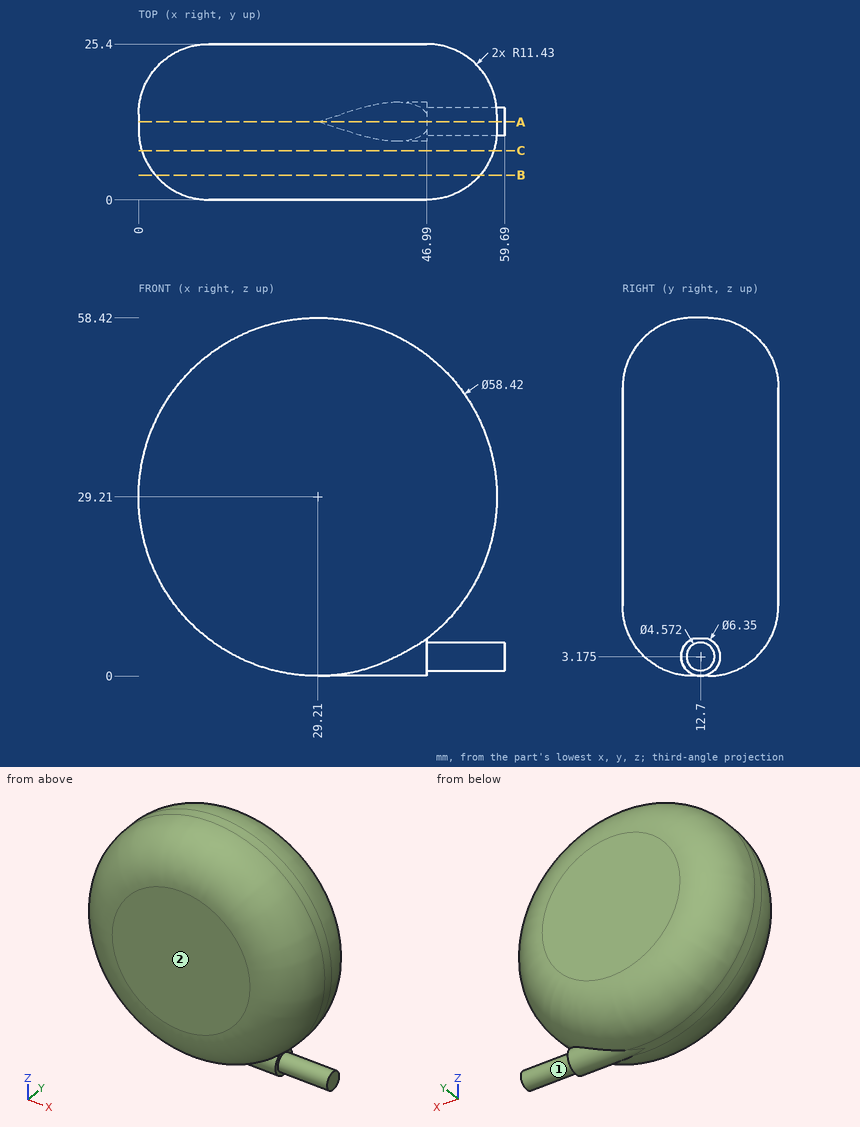
Part print with two shaded views. Sizes in mm from the minimum x, y, z corner. Give positions to 0.01 mm unless a question says otherwise; leave off trailing zeros. Order: outer loops, then holes, each group sorted by start corner. A loop starts at its lowest first (then second) coordinate and runs counter-clockwise, first axis right, second up. Notation, with made-up numbers: (-12.5, 3.25) - (21.5, 3.25) arc R16 cw to (21.5, 14.25) - close; hole circle Ø1 at (58, 16). An arc over 180 degrees is marked (long way). Write each question's results on one line, items separated by ' | '.
1. Saw through at A-A on y = 12.7. List the corners of the cut face in (x, z).
Calculated:
outline: (29.21, 0) - (46.99, 0) - (46.99, 0.89) - (59.69, 0.89) - (59.69, 5.46) - (46.99, 5.46) - (46.99, 6.03) arc R29.21 ccw (long way) to start
2. Saw through at C-C on y = 8. List the corners of the cut face in (x, z), and give its area (3 significant figures).
Calculated:
outline: circle Ø57.37 at (29.21, 29.21) | area: 2,580 mm2
3. Probe L1, parallel to Z at x = 9.5, y = 20.5; L2, parallel to Y at x = 32.5, z = 48.5; L3, parallel to Y at x = 25.5, z = 51. List the from-to ranges inside material, lowest first. Write a range as from..to.
Calculated:
L1: z = 10.52..47.9 | L2: y = 0.14..25.26 | L3: y = 0.85..24.55
4. Saw through at B-B on y = 4. List the corners of the cut face in (x, z), and give its area (3 significant figures).
Calculated:
outline: circle Ø52.93 at (29.21, 29.21) | area: 2,200 mm2
5. Pin check, flat tips, straight feed: pin 1 (4 mm diameter, centred on x = 32, y = 10, fed in from +Z); pin 2 (8 mm diameter, centred on y = 13, z = 47.5, fed in from -X); pin 3 (1 mm diameter, centred on y = 6, z = 41, fed in from -X). Stop position of each tip, or through.
Calculated:
pin 1: stops at z = 58.39 | pin 2: stops at x = 3.73 | pin 3: stops at x = 3.63
6. Pull direction Z, two halves, no side cores. Call the marked faces 1 and 2: released by +Z, released by -Z, zero draft, split by the parting line, or undercut.
Calculated:
face 1: undercut | face 2: zero draft
